The figure shows three views and two pictorial views of one solid part (mm, origin at its lowest corner). Answer the questions. Give positions to 0.01 mm unless a question says otherwise; leave off trailing zeros. Order: outer loops, then holes, each group sorted by start corner. A loop starts at its lowest first (then second) coordinate and runs counter-clockwise, first axis right, second up. Notation, with made-up numbers: (24.5, 40) - (59.5, 40) arc R28 cw to (59.5, 71) - close; hole circle Ø3 at (1, 21). An arc over 180 degrees is marked (long way). Answer as a JSON object with one key per item and string values. Group by question number.
Q1. A cutting plane is placed at B-B, the plane z = 64.5. Give the vertices of the cut face in (x, y).
Q2. A cutting plane is placed at A-A, the plane y = 3. Count the separate pieces of the cut face and the enclosed holes in it, and give its area (3 significant figures).
Q3. A cutting plane is placed at C-C, the plane x = 12. Give the vertices of the cut face in (y, z), and give its area (3 significant figures).
Q4. Consider line 1 (X direction, y = 5.75, z = 20); line 2 (X direction, y = 6.25, z = 30.5); line 3 (Z direction, x = 106.5, y = 0.5). Determine where each line is inside the solid, lowest interval first.
Q5. Given pin 1 (3 mm diameter, centred on y = 3.5, z = 123, fed in from -X); pin 2 (1.9 mm diameter, centred on y = 3, z = 2, fed in from +X); pin 3 (1.9 mm diameter, centred on x = 110, y = 4.5, fed in from +Z); pin 4 (3 mm diameter, centred on x = 102.235, z = 20.955, fed in from +Y), each flat-ended and moving along its own axis, determine where each tip first touches the part or whether it passes through.
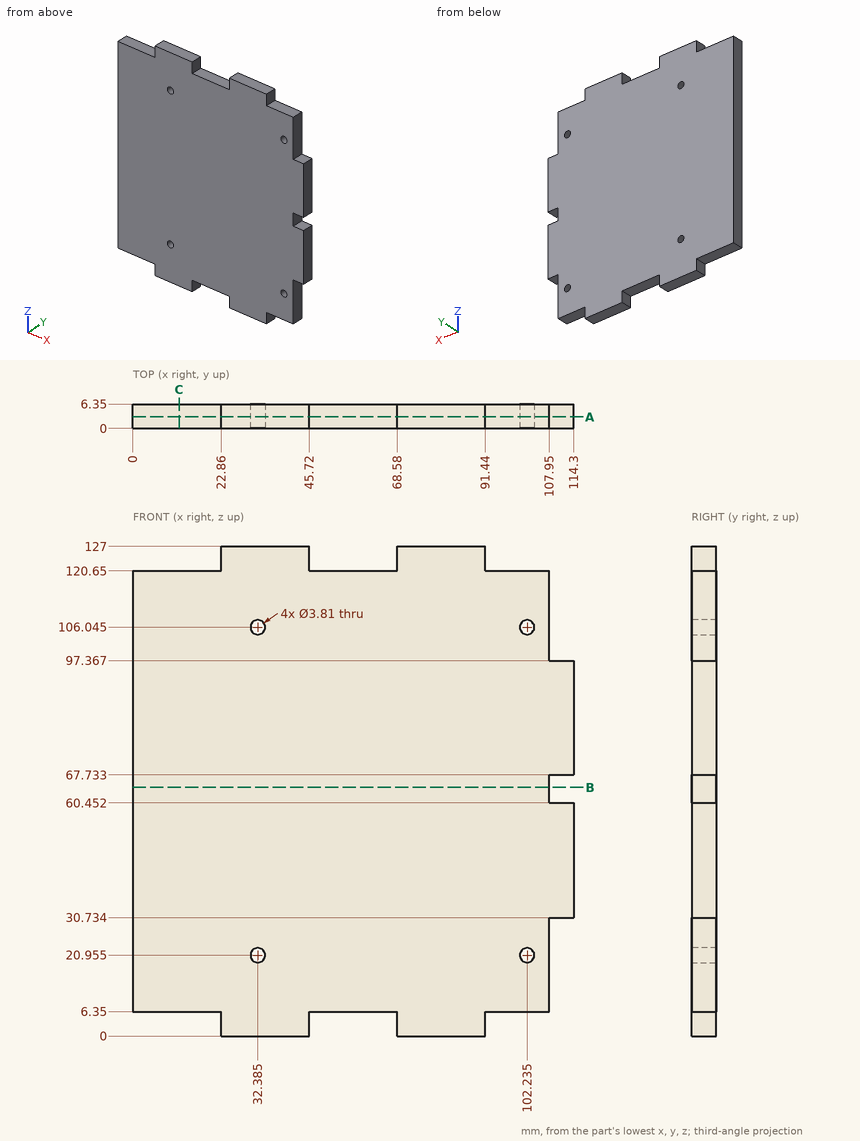
Reply:
{
 "1": {"outline": "(0, 0) - (107.95, 0) - (107.95, 6.35) - (0, 6.35) - close"},
 "2": {"separate pieces": "1", "enclosed holes": "4", "area": "13,300 mm^2"},
 "3": {"outline": "(0, 6.35) - (6.35, 6.35) - (6.35, 120.65) - (0, 120.65) - close", "area": "726 mm^2"},
 "4": {"line 1": "x = 0 to 30.74, 34.03 to 100.59, 103.88 to 107.95", "line 2": "x = 0 to 107.95", "line 3": "z = 6.35 to 120.65"},
 "5": {"pin 1": "stops at x = 22.86", "pin 2": "stops at x = 91.44", "pin 3": "stops at z = 97.37", "pin 4": "passes through"}
}
